Read the model definition and answer for the solid it produces. Units are mm, in the model's axes. A direction names the side the tool comes from. Coordinates: 2 decimals unless noted, no trailing zeros. Loops run counter-clockwise (first coordinate to the right, second up) from the corner with the lowest first, then second, coordinate; pieces in that order, holes last. Notation, with made-up numbers: M 70.25,16.25 L 97.25,16.25 A20 ccw 97.25,33.25 Z; hole C 68.25,13.25 d8. An arc over 180 degrees is marked long. Put each result on its own line as item: value.
from build123d import *

# Parameters (mm, degrees)
F0_R      = 50.8
F1_DEPTH  = 25.4
F2_R      = 12.7
F3_R      = 7.62
F5_DEPTH  = 304.8
F4_R      = 7.62
F6_DEPTH  = 304.8
F8_R      = 50.8
F9_DEPTH  = 25.4
F10_R     = 12.7
F11_R     = 12.69999
F9_FACE_R = 38.10001
F22_R     = 12.7
F24_R     = 5.08


# Not quite as in the source:
# - a fillet or chamfer is up to 0.001 mm smaller than in the source, because OpenCascade refuses the exact size
# - the program builds the solid bodies; features that only make, move or delete a surface that nothing else refers to are left out


with BuildPart() as f1:
    # F0 (on Top) → F1 (new body)
    with BuildSketch(Plane.XY):
        Circle(F0_R)
    extrude(amount=F1_DEPTH)

    # F2
    f2_edges = [f1.edges().sort_by_distance(p)[0] for p in [
        (-50.8, 0, 25.4),
    ]]
    fillet(f2_edges, radius=F2_R)

    # F3 (on face) → F5 (join)
    with BuildSketch(Plane.XY.offset(25.4)):
        with Locations((-17.3765644431, 14.6533707157)):
            Circle(F3_R)
    extrude(amount=F5_DEPTH)

    # F4 (on face) → F6 (join)
    with BuildSketch(Plane.XY.offset(25.4)):
        with Locations((15.8204566687, 14.3940197304)):
            Circle(F4_R)
        with Locations((15.8195672557, -12.837909162)):
            Circle(F4_R)
        with Locations((-17.1172115952, -12.837909162)):
            Circle(F4_R)
    extrude(amount=F6_DEPTH)

    # F8 (on offset) → F9 (join)
    with BuildSketch(Plane.XY.offset(330.2)):
        Circle(F8_R)
    extrude(amount=F9_DEPTH)

    # F10
    f10_edges = [f1.edges().sort_by_distance(p)[0] for p in [
        (-50.8, 0, 330.2),
    ]]
    fillet(f10_edges, radius=F10_R)

    # F11 (radius 12.7 in the source; OpenCascade refuses exactly that, so slightly less here)
    f11_edges = [f1.edges().sort_by_distance(p)[0] for p in [
        (-50.8, 0, 355.6),
    ]]
    fillet(f11_edges, radius=F11_R)

    # F9_face (on face) → F23 section 0
    with BuildSketch(Plane.XY.offset(355.6)):
        Circle(F9_FACE_R)
    # F22 (on offset) → F23 section 1
    with BuildSketch(Plane.XY.offset(393.7)):
        Circle(F22_R)
    loft()

    # F24
    f24_edges = [f1.edges().sort_by_distance(p)[0] for p in [
        (-12.7, 0, 393.7),
    ]]
    fillet(f24_edges, radius=F24_R)


solid = f1.part
1) Find section B-B, the plane z = 71. Write down the section's boundary in (x, y).
Answer list:
outline: C -17.38,14.65 d15.24; C -17.12,-12.84 d15.24; C 15.82,-12.84 d15.24; C 15.82,14.39 d15.24
2) Straight lines are drawn through the part: line 1 (Z direction, x = 2, y = -9.5); line 2 (Y direction, x = 16.5, z = 77); line 3 (Z direction, x = 39.5, y = -15). For each, find the intervals that lie inside material, in ascending order. Write a range as [from, to].
Answer list:
line 1: z = [0, 25.4], [330.2, 393.7]
line 2: y = [-20.43, -5.25], [6.8, 21.98]
line 3: z = [0, 24.7], [330.9, 354.9]
3) Which of the six approach directions +Z, -Z, +X, -X, +Y, -Y give full straight-line access (tool end or side, diameter ignored) to faces 4 (the conical face through (17.19, 5.41, 385.72)), 5 (the cylindrical face through (14.828, -5.283, 175.666))?
Answer list:
face 4: +Z
face 5: none
4) Find section C-C, the plane z = 362. Write down the section's boundary in (x, y).
Answer list:
outline: C 0,0 d67.67
5) Given pin 1 Ø1.5 at (x, y) = (-38.5, 18.5) entering from +Z; pin 2 Ø1.5 at (y, z) = (-21.5, 212) entering from -X; pin 3 Ø12 at (y, z) = (-18, 96) entering from -X; pin 4 Ø12 at (y, z) = (7.5, 276.5) entering from -X, each flat-ended and moving along its own axis, determine where each tip first touches the part or whether it passes through.
Answer list:
pin 1: stops at z = 355
pin 2: passes through
pin 3: stops at x = -24.74
pin 4: stops at x = -24.91
6) Determine the mould class of faces 1 (the cylindrical face through (-13.021, -6.413, 175.666)), 2 (the flat face through (0, 0, 393.7)), 3 (the cylindrical face through (-11.012, -49.592, 6.261)) for opening direction Z: released by +Z, released by -Z, zero draft, split by the parting line, or undercut.
Answer list:
face 1: undercut
face 2: released by +Z
face 3: zero draft
